Geometry: final body of the model. Coordinates: model frame, mm. Face numbers are marked on the shaded views. A direction names the side the tool comes from. Give positions to 0.01 mm unless a question says otherwise; leave off trailing zeros. Order: outer loops, then holes, each group sorted by start corner. A loop starts at its lowest first (then second) coordinate and runs counter-clockwise, first axis right, second up. Notation, with made-up numbers: (54, -21.5) - (62, -21.5) arc R31 ccw to (62, 4.5) - close; hole circle Ø2 at (37, 29.5). An arc over 180 degrees is marked (long way). One line per item, written item: value.
```python
from build123d import *

# Parameters (mm, degrees)
SK_MAIN_EXTRUSION_R   = 3.4
SK_MAIN_EXTRUSION_R_2 = 9
MAIN_EXTRUSION_DEPTH  = 25


with BuildPart() as part:
    # Sk Main Extrusion → Main Extrusion (new body)
    with BuildSketch(Plane.XY):
        with BuildLine():
            Line((5.222054351, 27.806515107), (4.190076845, 24.971180212))
            ThreePointArc((4.190076845, 24.971180212), (4.175951325, 24.863886241), (4.208493649, 24.760675177))
            Line((4.208493649, 24.760675177), (4.987558066, 23.411296024))
            Line((4.987558066, 23.411296024), (5.718509166, 23.145251581))
            Line((5.718509166, 23.145251581), (8.396186179, 24.11984631))
            ThreePointArc((8.396186179, 24.11984631), (8.811074612, 24.086489799), (9.056960151, 23.750654467))
            ThreePointArc((9.056960151, 23.750654467), (8.933433013, 20.965882372), (7.504160339, 18.572684887))
            Line((7.504160339, 18.572684887), (6.540737726, 17.609262274))
            ThreePointArc((6.540737726, 17.609262274), (0, 14.9), (-6.540737726, 17.609262274))
            Line((-6.540737726, 17.609262274), (-7.504160339, 18.572684887))
            ThreePointArc((-7.504160339, 18.572684887), (-8.933433013, 20.965882372), (-9.056960151, 23.750654467))
            ThreePointArc((-9.056960151, 23.750654467), (-8.811074612, 24.086489799), (-8.396186179, 24.11984631))
            Line((-8.396186179, 24.11984631), (-5.718509166, 23.145251581))
            Line((-5.718509166, 23.145251581), (-4.987558066, 23.411296024))
            Line((-4.987558066, 23.411296024), (-4.208493649, 24.760675177))
            ThreePointArc((-4.208493649, 24.760675177), (-4.175951325, 24.863886241), (-4.190076845, 24.971180212))
            Line((-4.190076845, 24.971180212), (-5.222054351, 27.806515107))
            ThreePointArc((-5.222054351, 27.806515107), (-5.496641489, 28.164364033), (-5.926823816, 28.3))
            Line((-5.926823816, 28.3), (-20.591883092, 28.3))
            ThreePointArc((-20.591883092, 28.3), (-21.165908241, 28.185819299), (-21.652543264, 27.860660172))
            Line((-21.652543264, 27.860660172), (-48.436814511, 1.076388924))
            ThreePointArc((-48.436814511, 1.076388924), (-48.876154339, 0.015728753), (-48.436814511, -1.044931419))
            Line((-48.436814511, -1.044931419), (-35.355339059, -14.126406871))
            ThreePointArc((-35.355339059, -14.126406871), (0, -28.771067812), (35.355339059, -14.126406871))
            Line((35.355339059, -14.126406871), (48.436814511, -1.044931419))
            ThreePointArc((48.436814511, -1.044931419), (48.876154339, 0.015728753), (48.436814511, 1.076388924))
            Line((48.436814511, 1.076388924), (21.652543264, 27.860660172))
            ThreePointArc((21.652543264, 27.860660172), (21.165908241, 28.185819299), (20.591883092, 28.3))
            Line((20.591883092, 28.3), (5.926823816, 28.3))
            ThreePointArc((5.926823816, 28.3), (5.496641489, 28.164364033), (5.222054351, 27.806515107))
        make_face()
        with Locations((-18.106601718, 20.8)):
            Circle(SK_MAIN_EXTRUSION_R, mode=Mode.SUBTRACT)
        with Locations((18.106601718, 20.8)):
            Circle(SK_MAIN_EXTRUSION_R, mode=Mode.SUBTRACT)
        Circle(SK_MAIN_EXTRUSION_R_2, mode=Mode.SUBTRACT)
        with Locations((0, -19.1)):
            Circle(SK_MAIN_EXTRUSION_R, mode=Mode.SUBTRACT)
        with BuildLine():
            Line((33.410795411, -12.181863223), (43.025551853, -2.567106781))
            ThreePointArc((43.025551853, -2.567106781), (43.242324604, -1.477316568), (42.318445072, -0.86))
            Line((42.318445072, -0.86), (12.360841395, -0.86))
            ThreePointArc((12.360841395, -0.86), (11.708461138, -1.102108187), (11.371974084, -1.7112))
            ThreePointArc((11.371974084, -1.7112), (8.980737669, -7.183059997), (4.167977698, -10.718113729))
            ThreePointArc((4.167977698, -10.718113729), (2.911454942, -12.309920658), (3.692145622, -14.181609948))
            ThreePointArc((3.692145622, -14.181609948), (6.052344462, -18.008383533), (5.177787873, -22.418585955))
            ThreePointArc((5.177787873, -22.418585955), (5.184897798, -24.588029411), (7.164897408, -25.474673081))
            ThreePointArc((7.164897408, -25.474673081), (21.348803489, -20.923067641), (33.410795411, -12.181863223))
        make_face(mode=Mode.SUBTRACT)
        with BuildLine():
            Line((-12.360841395, -0.86), (-42.318445072, -0.86))
            ThreePointArc((-42.318445072, -0.86), (-43.242324604, -1.477316568), (-43.025551853, -2.567106781))
            Line((-43.025551853, -2.567106781), (-33.410795411, -12.181863223))
            ThreePointArc((-33.410795411, -12.181863223), (-21.348803489, -20.923067641), (-7.164897408, -25.474673081))
            ThreePointArc((-7.164897408, -25.474673081), (-5.184897798, -24.588029411), (-5.177787873, -22.418585955))
            ThreePointArc((-5.177787873, -22.418585955), (-6.052344462, -18.008383533), (-3.692145622, -14.181609948))
            ThreePointArc((-3.692145622, -14.181609948), (-2.911454942, -12.309920658), (-4.167977698, -10.718113729))
            ThreePointArc((-4.167977698, -10.718113729), (-8.980737669, -7.183059997), (-11.371974084, -1.7112))
            ThreePointArc((-11.371974084, -1.7112), (-11.708461138, -1.102108187), (-12.360841395, -0.86))
        make_face(mode=Mode.SUBTRACT)
        with BuildLine():
            Line((42.027009358, 3.597106781), (25.770007578, 19.854108561))
            ThreePointArc((25.770007578, 19.854108561), (24.790343945, 20.109141459), (24.089991835, 19.378190342))
            ThreePointArc((24.089991835, 19.378190342), (18.61547326, 14.671089024), (12.43962541, 18.410883107))
            ThreePointArc((12.43962541, 18.410883107), (11.559727537, 19.021544755), (10.632153091, 18.486069675))
            ThreePointArc((10.632153091, 18.486069675), (7.825100476, 14.952318837), (3.911288507, 12.705317448))
            ThreePointArc((3.911288507, 12.705317448), (3.237253104, 11.76683924), (3.898250879, 10.819133056))
            ThreePointArc((3.898250879, 10.819133056), (8.576111128, 7.661613271), (11.188421808, 2.6588))
            ThreePointArc((11.188421808, 2.6588), (11.541328052, 2.10539819), (12.161328052, 1.89))
            Line((12.161328052, 1.89), (41.319902577, 1.89))
            ThreePointArc((41.319902577, 1.89), (42.243782109, 2.507316568), (42.027009358, 3.597106781))
        make_face(mode=Mode.SUBTRACT)
        with BuildLine():
            Line((-25.770007578, 19.854108561), (-42.027009358, 3.597106781))
            ThreePointArc((-42.027009358, 3.597106781), (-42.243782109, 2.507316568), (-41.319902577, 1.89))
            Line((-41.319902577, 1.89), (-12.161328052, 1.89))
            ThreePointArc((-12.161328052, 1.89), (-11.541328052, 2.10539819), (-11.188421808, 2.6588))
            ThreePointArc((-11.188421808, 2.6588), (-8.576111128, 7.661613271), (-3.898250879, 10.819133056))
            ThreePointArc((-3.898250879, 10.819133056), (-3.237253104, 11.76683924), (-3.911288507, 12.705317448))
            ThreePointArc((-3.911288507, 12.705317448), (-7.825100476, 14.952318837), (-10.632153091, 18.486069675))
            ThreePointArc((-10.632153091, 18.486069675), (-11.559727537, 19.021544755), (-12.43962541, 18.410883107))
            ThreePointArc((-12.43962541, 18.410883107), (-18.61547326, 14.671089024), (-24.089991835, 19.378190342))
            ThreePointArc((-24.089991835, 19.378190342), (-24.790343945, 20.109141459), (-25.770007578, 19.854108561))
        make_face(mode=Mode.SUBTRACT)
    extrude(amount=-MAIN_EXTRUSION_DEPTH)


solid = part.part
```
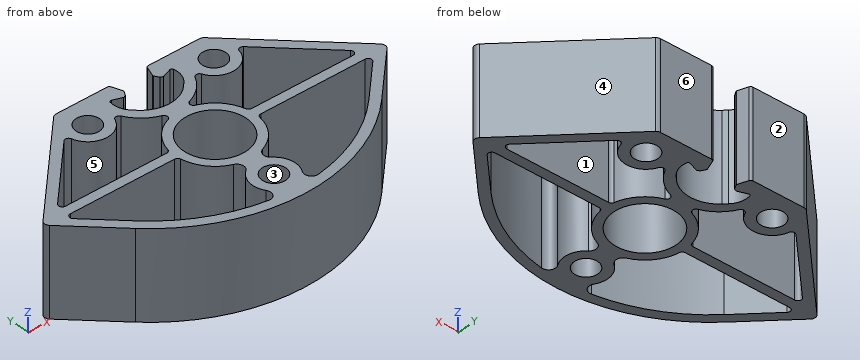
1) Section B-B, the plane y = -5.5. Return loops of the section in (x, z).
Answers below:
outline: (-43.98, -25) - (-40.09, -25) - (-40.09, 0) - (-43.98, 0) - close; (-10.1, -25) - (-7.12, -25) - (-7.12, 0) - (-10.1, 0) - close; (7.12, -25) - (10.1, -25) - (10.1, 0) - (7.12, 0) - close; (40.09, -25) - (43.98, -25) - (43.98, 0) - (40.09, 0) - close
2) Section D-D, the plane x = -28. Return loops of the section in (y, z).
Answers below:
outline: (-20.2, -25) - (-16.83, -25) - (-16.83, 0) - (-20.2, 0) - close; (-0.86, -25) - (1.89, -25) - (1.89, 0) - (-0.86, 0) - close; (17.62, -25) - (21.51, -25) - (21.51, 0) - (17.62, 0) - close
3) Section C-C, the plane x = -17.5. Return loops of the section in (y, z), then the cut area to 3 significant figures.
Answers below:
outline: (-25.61, -25) - (-22.66, -25) - (-22.66, 0) - (-25.61, 0) - close; (-0.86, -25) - (1.89, -25) - (1.89, 0) - (-0.86, 0) - close; (14.68, -25) - (17.45, -25) - (17.45, 0) - (14.68, 0) - close; (24.15, -25) - (28.3, -25) - (28.3, 0) - (24.15, 0) - close
area: 316 mm^2
4) First-contact query: pin 1 (5 mm diameter, centred on x = 13, z = -11.5, fed in from -Y); pin 2 (7.5 mm diameter, centred on x = 32, z = -7.5, fed in from -Y); pin 3 (8 mm diameter, centred on x = 18, z = -5.5, fed in from -Y). Flat tips, straight axial feed; report the tip coordinate or a pass-through.
Answers below:
pin 1: y = -27.66
pin 2: y = -20.03
pin 3: y = -26.77
5) Set-up query: the marked faces 1 and 2. Return all of +Z, -Z, +X, -X, +Y, -Y with unobstructed straight access to the full face (end or side cutting, diameter ignored); none if empty.
Answers below:
face 1: +Z, -Z
face 2: +Z, -Z, +X, -X, +Y
6) Material intervals for line 1 along Y through (x, z) = (0, -10.5); line 2 along Y through (x, z) = (-29, -7.5); line 3 along Y through (x, z) = (20, -5.25), sorted ascending.
Answers below:
line 1: -28.77 to -22.5, -15.7 to -9, 9 to 14.9
line 2: -19.5 to -16.07, -0.86 to 1.89, 16.62 to 20.51
line 3: -24.6 to -21.58, -0.86 to 1.89, 14.95 to 17.98, 23.62 to 28.3
7) Section A-A, the plane x = 0. Return loops of the section in (y, z).
Answers below:
outline: (-28.77, -25) - (-22.5, -25) - (-22.5, 0) - (-28.77, 0) - close; (-15.7, -25) - (-9, -25) - (-9, 0) - (-15.7, 0) - close; (9, -25) - (14.9, -25) - (14.9, 0) - (9, 0) - close
8) Mould query, pull axis X, two halves, no side actions, for the marked faces 3, 4, 5 and 6. Classes: released by +X, released by -X, zero draft, split by the parting line, or undercut.
Answers below:
face 3: undercut
face 4: released by +X
face 5: undercut
face 6: zero draft
